from build123d import *

# Parameters (mm, degrees)
SKETCH1_W           = 19.558
SKETCH1_H           = 10.16
SKETCH1_W_2         = 0.6096
SKETCH1_H_2         = 4.064
BOSS_EXTRUDE1_DEPTH = 6.35
SKETCH2_R           = 1.27
CUT_EXTRUDE1_DEPTH  = 6.35
SKETCH1_4_W         = 0.3302
SKETCH1_4_H         = 1.143
BOSS_EXTRUDE2_DEPTH = 6.35


with BuildPart() as part:
    # Sketch1 → Boss-Extrude1 (new body)
    with BuildSketch(Plane(origin=(0, 0, 0), x_dir=(1, 0, 0), z_dir=(0, 1, 0))):
        with Locations((10.092764077, 6.29705611)):
            Rectangle(SKETCH1_W, SKETCH1_H)
        with Locations((2.142564077, -0.81494389)):
            Rectangle(SKETCH1_W_2, SKETCH1_H_2)
        with Locations((18.042964077, -0.81494389)):
            Rectangle(SKETCH1_W_2, SKETCH1_H_2)
        with Locations((10.397564077, -0.81494389)):
            Rectangle(SKETCH1_W_2, SKETCH1_H_2)
    extrude(amount=BOSS_EXTRUDE1_DEPTH)

    # Sketch2 → Cut-Extrude1 (cut)
    with BuildSketch(Plane(origin=(0, 6.35, 0), x_dir=(1, 0, 0), z_dir=(0, 1, 0))):
        with Locations((4.631764077, 3.858413602)):
            Circle(SKETCH2_R)
        with Locations((14.791764077, 3.858413602)):
            Circle(SKETCH2_R)
    extrude(amount=-CUT_EXTRUDE1_DEPTH, mode=Mode.SUBTRACT)

    # Sketch1<4> → Boss-Extrude2 (add)
    with BuildSketch(Plane(origin=(0, 0, 0), x_dir=(1, 0, 0), z_dir=(0, 1, 0))):
        with Locations((16.912664077, 11.94855611)):
            Rectangle(SKETCH1_4_W, SKETCH1_4_H)
        Polygon((16.747564077, 12.52005611), (17.077764077, 12.52005611), (17.077764077, 12.85025611), (3.869764077, 12.85025611), (3.869764077, 12.52005611), align=None)
    extrude(amount=BOSS_EXTRUDE2_DEPTH)


solid = part.part
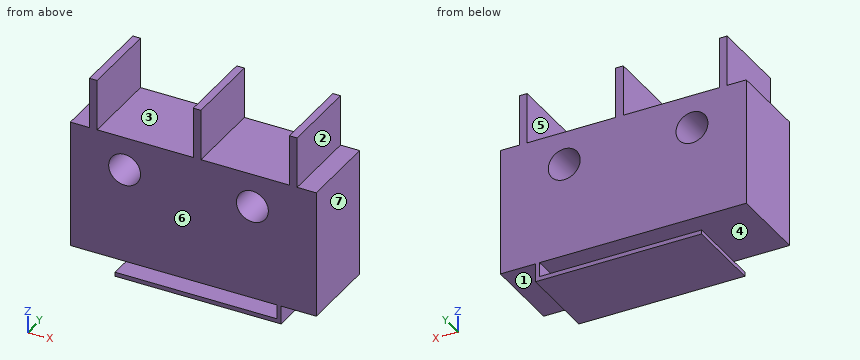
CAD build for the part. Positions are in the model's coordinates, mm. Face numbers are marked on the shaded views. A direction names the side the tool comes from. Round coordinates to 2 decimals unless told otherwise and drop trailing zeros. Loops run counter-clockwise (first coordinate to the right, second up) from the corner with the lowest first, then second, coordinate; pieces in that order, holes last.
(1) Drop flat-ended pins along their axis: pin 1 (0.9 mm diameter, centred on y = 2.5, z = -11.5, fed in from -X); pin 2 (2 mm diameter, centred on y = 2.5, z = 0, fed in from +X); pin 3 (1.2 mm diameter, centred on y = 3.5, z = 0, fed in from -X); pin 4 (3 mm diameter, centred on x = 7.5, y = 2.5, fed in from +Z). Give the stop position or say it passes through.
(2) Two-plate mould, pull along X, no slides. Class the marked faces 5, 6 and 7: +X half, -X half, draft (parallel to the pull), parting line (faces both ways), or undercut.
(3) Cut at A-A (x = 12). Give the cut face in (y, z).
(4) Which spindle directions (+Z, -Z, +X, -X, +Y, -Y) get a long thin tool onto all of the face, cutting with end or side? Do the marked faces 1, 2, 3 and 4. Say none if no direction does.
(5) Cut at D-D (y = 4.75). Give the cut face in (x, z), plus the area to 3 significant figures.
(6) Cut at C-C (x = 5). Give the cut face in (y, z), plus the area to 3 significant figures.
(7) Wall check: line 1 along X through (y, z) = (2.75, 1.5); line 2 along Z through (x, y) = (5, 1.5); line 3 along X through (y, z) = (6, -3.75). Give the ranges that are in metal, low to high.
(8) Cut at B-B (z = 0.5). Give the cut face in (x, y), plus the area to 3 significant figures.
Findings below:
1. pin 1: stops at x = 0.31
1. pin 2: stops at x = 18.35
1. pin 3: stops at x = 1.84
1. pin 4: stops at z = -1.22
2. face 5: undercut
2. face 6: draft
2. face 7: +X half
3. outline: (0, -12.85) - (6.35, -12.85) - (6.35, -12.52) - (0, -12.52) - close; (0, -11.38) - (6.35, -11.38) - (6.35, -1.22) - (0, -1.22) - close
4. face 1: -Z, +X, +Y, -Y
4. face 2: +Z, +X, +Y, -Y
4. face 3: +Z, +Y, -Y
4. face 4: -X, +Y, -Y
5. outline: (0.31, -11.38) - (16.75, -11.38) - (16.75, -12.52) - (3.87, -12.52) - (3.87, -12.85) - (17.08, -12.85) - (17.08, -11.38) - (19.87, -11.38) - (19.87, -1.22) - (18.35, -1.22) - (18.35, 2.85) - (17.74, 2.85) - (17.74, -1.22) - (10.7, -1.22) - (10.7, 2.85) - (10.09, 2.85) - (10.09, -1.22) - (2.45, -1.22) - (2.45, 2.85) - (1.84, 2.85) - (1.84, -1.22) - (0.31, -1.22) - close; hole circle Ø2.54 at (4.63, -3.86); hole circle Ø2.54 at (14.79, -3.86)
5. area: 201 mm2
6. outline: (0, -12.85) - (6.35, -12.85) - (6.35, -12.52) - (0, -12.52) - close; (0, -11.38) - (6.35, -11.38) - (6.35, -5.07) - (0, -5.07) - close; (0, -2.64) - (6.35, -2.64) - (6.35, -1.22) - (0, -1.22) - close
6. area: 51.2 mm2
7. line 1: x = 1.84 to 2.45, 10.09 to 10.7, 17.74 to 18.35
7. line 2: z = -12.85 to -12.52, -11.38 to -5.07, -2.64 to -1.22
7. line 3: x = 0.31 to 3.37, 5.9 to 13.53, 16.06 to 19.87
8. outline: (1.84, 0) - (2.45, 0) - (2.45, 6.35) - (1.84, 6.35) - close; (10.09, 0) - (10.7, 0) - (10.7, 6.35) - (10.09, 6.35) - close; (17.74, 0) - (18.35, 0) - (18.35, 6.35) - (17.74, 6.35) - close
8. area: 11.6 mm2
